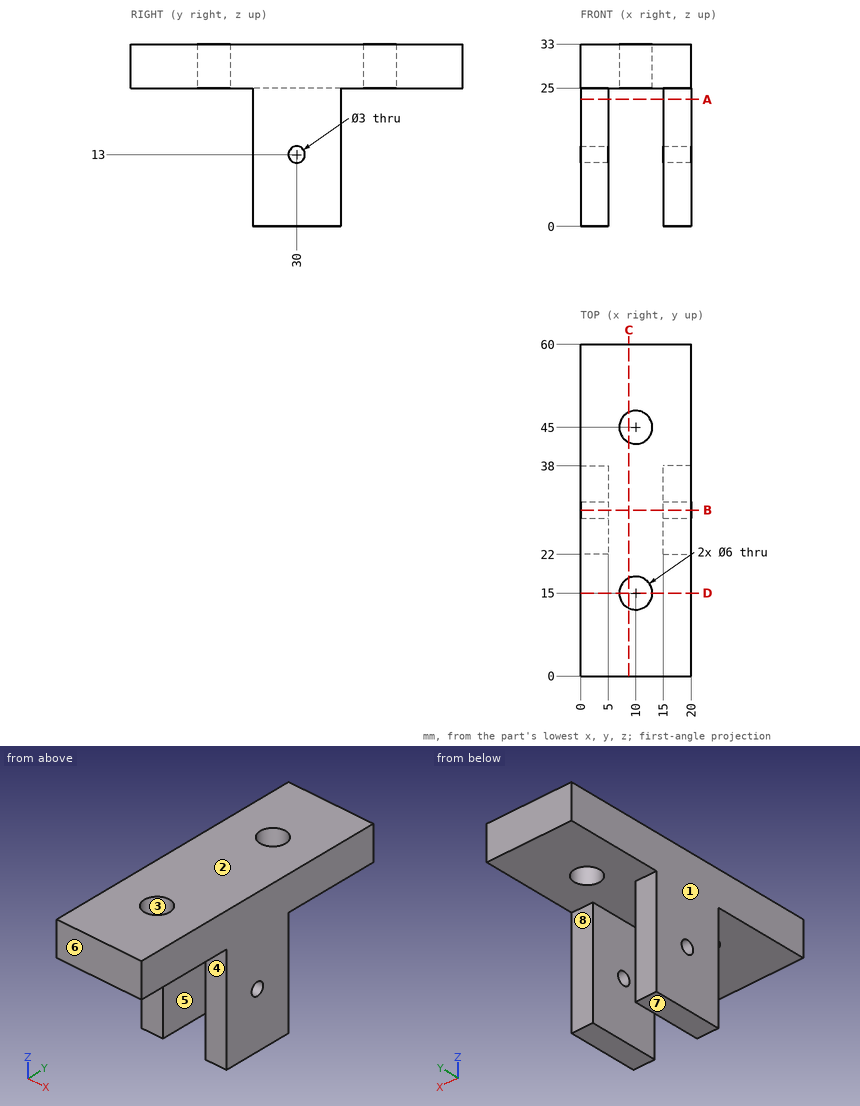
Source: three-view drawing plus pictorial views. Frame: mm from the lowest corner of the part. A direction names the side the tool comes from. Give positions to 0.01 mm unless a question says otherwise; leave off trailing zeros. Order: outer loops, then holes, each group sorted by start corner. A loop starts at its lowest first (then second) coordinate and runs counter-clockwise, first axis right, second up. Notation, with made-up numbers: M 7,45.5 L 63,45.5 A20 ccw 63,76.5 Z; hole C 13.25,80 d7. An arc over 180 degrees is marked long. Return JSON: item names as keys, results as strings.
1) Mould query, pull axis X, two halves, no side actions, for the marked faces 1, 2 and 3. Classes: released by +X, released by -X, zero draft, split by the parting line, or undercut.
Taken from the geometry:
{"face 1": "released by -X", "face 2": "zero draft", "face 3": "undercut"}
2) Line query: L1, parallel to Y at x = 10, z = 27.5; L2, parallel to X at y = 23.5, z = 5; L3, parallel to Z at x = 10.5, y = 6.5. Output: solid intervals per line, ascending. Write a range as [from, to].
Taken from the geometry:
{"L1": "y = [0, 12], [18, 42], [48, 60]", "L2": "x = [0, 5], [15, 20]", "L3": "z = [25, 33]"}
3) Section query C-C on x = 8.75. Output: boundary loops of the cut face in (y, z), and give its area (3 significant figures).
Taken from the geometry:
{"outline": "M 0,25 L 12.27,25 L 12.27,33 L 0,33 Z; M 17.73,25 L 42.27,25 L 42.27,33 L 17.73,33 Z; M 47.73,25 L 60,25 L 60,33 L 47.73,33 Z", "area": "393 mm2"}
4) Section query A-A on z = 23. Output: boundary loops of the cut face in (x, y), and give its area (3 significant figures).
Taken from the geometry:
{"outline": "M 0,22 L 5,22 L 5,38 L 0,38 Z; M 15,22 L 20,22 L 20,38 L 15,38 Z", "area": "160 mm2"}
5) Section query B-B on y = 30. Output: boundary loops of the cut face in (x, z).
Taken from the geometry:
{"outline": "M 0,0 L 5,0 L 5,11.5 L 0,11.5 Z; M 0,14.5 L 5,14.5 L 5,25 L 15,25 L 15,14.5 L 20,14.5 L 20,33 L 0,33 Z; M 15,0 L 20,0 L 20,11.5 L 15,11.5 Z"}
6) Section query D-D on y = 15. Output: boundary loops of the cut face in (x, z), and give its area (3 significant figures).
Taken from the geometry:
{"outline": "M 0,25 L 7,25 L 7,33 L 0,33 Z; M 13,25 L 20,25 L 20,33 L 13,33 Z", "area": "112 mm2"}
7) Contact query for flat-ended pins moving along their axis: pin 1 (2 mm diameter, centred on x = 9, y = 19.5, fed in from -Z); pin 2 (1.5 mm diameter, centred on x = 17.5, z = 7, fed in from -Y); pin 3 (2 mm diameter, centred on y = 39.5, z = 16.5, fed in from -X); pin 4 (10 mm diameter, centred on x = 9.5, z = 10, fed in from +Y). Output: stop coordinate, or through.
Taken from the geometry:
{"pin 1": "stops at z = 25", "pin 2": "stops at y = 22", "pin 3": "passes through", "pin 4": "stops at y = 38"}
8) Access query for the marked faces 4, 5, 6, 7 and 8. Directions: +Z, -Z, +X, -X, +Y, -Y. A direction counts if a zero-diameter tool reaches every point of the face in a straight line with its end or side. Return the directions, or none.
Taken from the geometry:
{"face 4": "-Z, +X, -X, -Y", "face 5": "-Z, +Y, -Y", "face 6": "+Z, -Z, +X, -X, -Y", "face 7": "-Z, +X, -X, +Y, -Y", "face 8": "-Z, +X, -X, +Y"}
